```python
from build123d import *

# Parameters (mm, degrees)
SKETCH2_W                                           = 1073.15
SKETCH2_H                                           = 1073.15
BOSS_EXTRUDE2_DEPTH                                 = 152.4
SKETCH6_W                                           = 1054.1
SKETCH6_H                                           = 1054.1
CUT_EXTRUDE3_DEPTH                                  = 142.875
SKETCH7_W                                           = 768.35
SKETCH7_H                                           = 768.35
CUT_EXTRUDE4_DEPTH                                  = 142.875
SKETCH8_R                                           = 3.5687
CUT_EXTRUDE5_DEPTH                                  = 1270
SKETCH9_R                                           = 2.50063
CUT_EXTRUDE6_DEPTH                                  = 1270
CUT_EXTRUDE7_DEPTH                                  = 1016
CUT_EXTRUDE8_DEPTH                                  = 154.94
CUT_EXTRUDE8_DEPTH_BACK                             = 10.16
CSK_FOR_1_4_FLAT_HEAD_MACHINE_SCREW_100_D           = 6.7564
CSK_FOR_1_4_FLAT_HEAD_MACHINE_SCREW_100_CSINK_D     = 16.510254
CSK_FOR_1_4_FLAT_HEAD_MACHINE_SCREW_100_CSINK_ANGLE = 100
CSK_FOR_1_4_FLAT_HEAD_MACHINE_SCREW_2_D             = 6.7564
CSK_FOR_1_4_FLAT_HEAD_MACHINE_SCREW_2_CSINK_D       = 16.510254
CSK_FOR_1_4_FLAT_HEAD_MACHINE_SCREW_2_CSINK_ANGLE   = 100
CSK_FOR_1_4_FLAT_HEAD_MACHINE_SCREW_3_D             = 6.7564
CSK_FOR_1_4_FLAT_HEAD_MACHINE_SCREW_3_CSINK_D       = 16.510254
CSK_FOR_1_4_FLAT_HEAD_MACHINE_SCREW_3_CSINK_ANGLE   = 100
CSK_FOR_1_4_FLAT_HEAD_MACHINE_SCREW_4_D             = 6.7564
CSK_FOR_1_4_FLAT_HEAD_MACHINE_SCREW_4_CSINK_D       = 16.510254
CSK_FOR_1_4_FLAT_HEAD_MACHINE_SCREW_4_CSINK_ANGLE   = 100


with BuildPart() as part:
    # Sketch2 → Boss-Extrude2 (new body)
    with BuildSketch(Plane(origin=(0, 0, 0), x_dir=(1, 0, 0), z_dir=(0, 1, 0))):
        with Locations((-30.964668371, 76.000745145)):
            Rectangle(SKETCH2_W, SKETCH2_H)
    extrude(amount=BOSS_EXTRUDE2_DEPTH)

    # Sketch6 → Cut-Extrude3 (cut)
    with BuildSketch(Plane(origin=(0, 152.4, 0), x_dir=(1, 0, 0), z_dir=(0, 1, 0))):
        with Locations((-30.964668371, 76.000745145)):
            Rectangle(SKETCH6_W, SKETCH6_H)
    extrude(amount=-CUT_EXTRUDE3_DEPTH, mode=Mode.SUBTRACT)

    # Sketch7 → Cut-Extrude4 (cut)
    with BuildSketch(Plane(origin=(0, 9.525, 0), x_dir=(1, 0, 0), z_dir=(0, 1, 0))):
        with Locations((-30.964668371, 76.000745145)):
            Rectangle(SKETCH7_W, SKETCH7_H)
    extrude(amount=-CUT_EXTRUDE4_DEPTH, mode=Mode.SUBTRACT)

    # Sketch8 → Cut-Extrude5 (cut)
    with BuildSketch(Plane.XY.offset(460.574254855)):
        with Locations((273.835331629, 114.3)):
            Circle(SKETCH8_R)
        with Locations((70.635331629, 114.3)):
            Circle(SKETCH8_R)
        with Locations((-132.564668371, 114.3)):
            Circle(SKETCH8_R)
        with Locations((-335.764668371, 114.3)):
            Circle(SKETCH8_R)
    extrude(amount=-CUT_EXTRUDE5_DEPTH, mode=Mode.SUBTRACT)

    # Sketch9 → Cut-Extrude6 (cut)
    with BuildSketch(Plane.ZY.offset(567.539668371)):
        with Locations((295.474254855, 114.3)):
            Circle(SKETCH9_R)
        with Locations((146.884254855, 114.3)):
            Circle(SKETCH9_R)
        with Locations((-1.705745145, 114.3)):
            Circle(SKETCH9_R)
        with Locations((-150.295745145, 114.3)):
            Circle(SKETCH9_R)
        with Locations((-298.885745145, 114.3)):
            Circle(SKETCH9_R)
        with Locations((-447.475745145, 114.3)):
            Circle(SKETCH9_R)
    extrude(amount=-CUT_EXTRUDE6_DEPTH, mode=Mode.SUBTRACT)

    # Sketch10 → Cut-Extrude7 (cut)
    with BuildSketch(Plane.XZ):
        Polygon((-415.139668371, -460.175745145), (-415.139668371, 308.174254855), (-567.539668371, 460.574254855), (-567.539668371, -612.575745145), (505.610331629, -612.575745145), (505.610331629, 460.574254855), (353.210331629, 308.174254855), (353.210331629, -460.175745145), align=None)
    extrude(amount=-CUT_EXTRUDE7_DEPTH, mode=Mode.SUBTRACT)

    # Sketch11 → Cut-Extrude8 (cut, two sides: drawn at the far end of the back side and taken through both)
    with BuildSketch(Plane(origin=(0, 9.525, 0), x_dir=(1, 0, 0), z_dir=(0, 1, 0)).offset(-CUT_EXTRUDE8_DEPTH_BACK)):
        Polygon((-567.539668371, -460.574254855), (-558.014668371, -451.049254855), (-558.014668371, -460.574254855), align=None)
        Polygon((496.085331629, -451.049254855), (505.610331629, -460.574254855), (496.085331629, -460.574254855), align=None)
    extrude(amount=CUT_EXTRUDE8_DEPTH + CUT_EXTRUDE8_DEPTH_BACK, mode=Mode.SUBTRACT)

    # CSK for 1_4 Flat Head Machine Screw _100 (through all)
    with Locations(Plane(origin=(273.835331629, 114.3, 451.049254855), x_dir=(-1, 0, 0), z_dir=(0, 0, -1))):
        with Locations((0, 0)):
            CounterSinkHole(CSK_FOR_1_4_FLAT_HEAD_MACHINE_SCREW_100_D / 2, CSK_FOR_1_4_FLAT_HEAD_MACHINE_SCREW_100_CSINK_D / 2, counter_sink_angle=CSK_FOR_1_4_FLAT_HEAD_MACHINE_SCREW_100_CSINK_ANGLE)

    # CSK for 1_4 Flat Head Machine Screw  2 (through all)
    with Locations(Plane(origin=(70.635331629, 114.3, 451.049254855), x_dir=(-1, 0, 0), z_dir=(0, 0, -1))):
        with Locations((0, 0)):
            CounterSinkHole(CSK_FOR_1_4_FLAT_HEAD_MACHINE_SCREW_2_D / 2, CSK_FOR_1_4_FLAT_HEAD_MACHINE_SCREW_2_CSINK_D / 2, counter_sink_angle=CSK_FOR_1_4_FLAT_HEAD_MACHINE_SCREW_2_CSINK_ANGLE)

    # CSK for 1_4 Flat Head Machine Screw  3 (through all)
    with Locations(Plane(origin=(-132.564668371, 114.3, 451.049254855), x_dir=(-1, 0, 0), z_dir=(0, 0, -1))):
        with Locations((0, 0)):
            CounterSinkHole(CSK_FOR_1_4_FLAT_HEAD_MACHINE_SCREW_3_D / 2, CSK_FOR_1_4_FLAT_HEAD_MACHINE_SCREW_3_CSINK_D / 2, counter_sink_angle=CSK_FOR_1_4_FLAT_HEAD_MACHINE_SCREW_3_CSINK_ANGLE)

    # CSK for 1_4 Flat Head Machine Screw  4 (through all)
    with Locations(Plane(origin=(-335.764668371, 114.3, 451.049254855), x_dir=(-1, 0, 0), z_dir=(0, 0, -1))):
        with Locations((0, 0)):
            CounterSinkHole(CSK_FOR_1_4_FLAT_HEAD_MACHINE_SCREW_4_D / 2, CSK_FOR_1_4_FLAT_HEAD_MACHINE_SCREW_4_CSINK_D / 2, counter_sink_angle=CSK_FOR_1_4_FLAT_HEAD_MACHINE_SCREW_4_CSINK_ANGLE)


solid = part.part
```
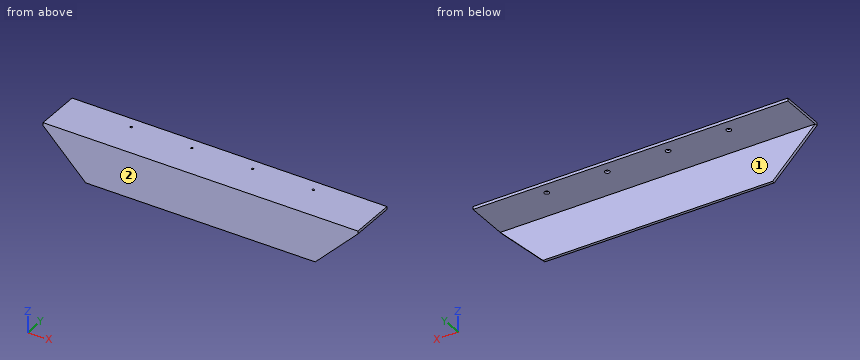
Geometry check sheet. Reference: the model listing, model coordinates, mm. Face numbers are marked on the shaded views. A direction names the side the tool comes from. Coordinates: 2 decimals unless noted, no trailing zeros. Order: outer loops, then holes, each group sorted by start corner. A loop starts at its lowest first (then second) coordinate and runs counter-clockwise, first axis right, second up. Notation, with made-up numbers: (56.25, 65.25) - (111.25, 65.25) arc R14 cw to (111.25, 84.25) - close; hole circle Ø8 at (33.25, -38.75). An arc over 180 degrees is marked (long way). Answer in a Markdown table with one row per item. Add a question column.
1. Section check B-B (z = 416). Enter the section's corners in (x, y) (3 decimals).
2. Section check C-C (y = 78). Enter the section's corners in (x, z), plus the area to 3 significant figures.
3. Gauge pin test, flat ends, axial feed: pin 1 Ø2 at (x, y) = (-294.5, 29.5) entering from -Z; pin 2 Ø9.5 at (x, y) = (-132.56, 114.3) entering from -Z. Record the tip position at first contact, or that the pin passes through.
4. Material ranges on L1, parallel to X at y = 114, z = 457; L2, parallel to Y at x = 179, z = 318 (3 decimals); L3, parallel to Z at x = 4, y = 99, recorded low to high. Write a range as [from, to].
5. Access from +Z, -Z, +X, -X, +Y, -Y to the whole of each face (thin tool, end or side, straight path). Record for the marked faces 1 and 2.
6. Section check D-D (x = -488). Enter the section's corners in (y, z) (3 decimals).
7. Section check A-A (x = -211.5). Enter the section's corners in (y, z) (3 decimals).
Data:
| question | item | result |
|---|---|---|
| 1 | outline | (-522.965, 0) - (461.036, 0) - (461.036, 9.525) - (-522.965, 9.525) - close |
| 2 | outline | (-558.01, 451.05) - (496.09, 451.05) - (496.09, 460.57) - (-558.01, 460.57) - close |
| 2 | area | 10,000 mm² |
| 3 | pin 1 | stops at z = 451.05 |
| 3 | pin 2 | stops at z = 453.99 |
| 4 | L1 | x = [-558.01, -339.32], [-332.21, -136.12], [-129.01, 67.08], [74.19, 270.28], [277.39, 496.09] |
| 4 | L2 | y = [0, 9.525] |
| 4 | L3 | z = [451.05, 460.57] |
| 5 | face 1 | -Z, +X, -X, +Y |
| 5 | face 2 | +Z, -Z, +X, -X, -Y |
| 6 | outline | (0, 381.035) - (9.525, 381.035) - (9.525, 451.049) - (152.4, 451.049) - (152.4, 460.574) - (0, 460.574) - close |
| 7 | outline | (0, 308.174) - (9.525, 308.174) - (9.525, 451.049) - (152.4, 451.049) - (152.4, 460.574) - (0, 460.574) - close |
